Autodesk Inventor part; units mm, degrees
ref_plane "YZ Plane" through (0, 0, 0) normal (1, 0, 0) x (0, 1, 0)
ref_plane "XZ Plane" through (0, 0, 0) normal (0, 1, 0) x (-1, 0, 0)
ref_plane "XY Plane" through (0, 0, 0) normal (0, 0, 1) x (1, 0, 0)
sketch "Sketch1" plane through (0, 0, 0) normal (0, 0, 1) x (1, 0, 0)
  line L0 (0, 0) -> (-110.8614, 0)
  line L1 (-110.8614, 0) -> (-110.8614, -1490)
  line L2 (-110.8614, -1490) -> (0, -1490)
  line L3 (0, -1490) -> (0, 0)
  line L4 (-110.8614, -1390) -> (-66, -1390)
  line L5 (-66, -1390) -> (-66, -1385)
  line L6 (-66, -1385) -> (-110.8614, -1385)
  line L7 (-110.8614, -1385) -> (-110.8614, -1390)
  line L8 (-110.8614, -893.3333) -> (-66, -893.3333)
  line L9 (-66, -893.3333) -> (-66, -888.3333)
  line L10 (-66, -888.3333) -> (-110.8614, -888.3333)
  line L11 (-110.8614, -888.3333) -> (-110.8614, -893.3333)
  line L12 (-110.8614, -396.6667) -> (-66, -396.6667)
  line L13 (-66, -396.6667) -> (-66, -391.6667)
  line L14 (-66, -391.6667) -> (-110.8614, -391.6667)
  line L15 (-110.8614, -391.6667) -> (-110.8614, -396.6667)
  circle A0 centre (-110.8614, -155) radius 30
  point P0 (-110.8614, -1385)
  point P1 (-110.8614, -125)
  point P2 (-110.8614, -185)
  dimension "d0" = 1490
  dimension "d1" = 110.8614
  dimension "d2" = 5
  dimension "d4" = 100
  dimension "d7" = 496.6667
  dimension "d23" = 66
  dimension "d28" = 60
  dimension "d29" = 1335
extrude "Plate1" add sketch "Sketch1" along normal blind 4 contours L3 L2 L1 L4 L5 L6 L8 L9 L10 L12 L13 L14 A0 L0
sketch "Sketch2" plane through (4, 0, 0) normal (-1, 0, 0) x (0, -1, 0)
  line L0 (1490, 0) -> (0, 0)
  line L1 (0, 0) -> (0, 60)
  line L2 (0, 60) -> (1490, 60)
  line L3 (1490, 60) -> (1490, 0)
edge flange "Flange1" height 60 angle 90 thickness 4 bend radius 4 thickness toward (-1, 0, 0) relief tear relief width 4 relief depth 2 edges at (0, -745, 4) wall of the first edge with corners at (4, -1490, 0) (4, 0, 0) (4, 0, 60) (4, -1490, 60)
bend "Bend1"
corner "Corner1"
chamfer "Corner Chamfer1" distance 3 angle 45 6 edges at (-110.8614, -1390, 2) (-110.8614, -1385, 2) (-110.8614, -893.3333, 2) (-110.8614, -888.3333, 2) (-110.8614, -391.6667, 2) (-110.8614, -396.6667, 2)
equation "\"d0\" = Стрингер_длина"
equation "\"d1\" = стрингер_глубина_8"
equation "\"d2\" = паз_под_стрингер_толщина"
equation "\"d7\" = 0.333333 * Стрингер_длина"
equation "\"d23\" = паз_под_стрингер_глубина - Thickness"
equation "\"d28\" = 2 * радиус_выреза_под_сварку"
equation "\"d12\" = Thickness"
equation "\"d13\" = BendReliefWidth"
equation "\"d14\" = BendReliefDepth"
equation "\"d15\" = MinimumRemnant"
equation "\"d16\" = TransitionRadius"
equation "\"d17\" = ребро_усилителей"
equation "\"d19\" = BendRadius"
equation "\"d20\" = CornerReliefSize"
equation "\"d21\" = GapSize"
equation "\"d22\" = JacobiRadiusSize"
equation "\"BendRadius\" = Thickness"
equation "\"BendReliefWidth\" = Thickness"
equation "\"BendReliefDepth\" = 0.5 * Thickness"
equation "\"CornerReliefSize\" = 4 * Thickness"
equation "\"MinimumRemnant\" = 2 * Thickness"
equation "\"TransitionRadius\" = BendRadius"
equation "\"JacobiRadiusSize\" = BendRadius"
equation "\"GapSize\" = Thickness"
properties part number "0382 GBK stringer 8" material "Steel"
The model under review builds one solid part; all positions refer to its coordinate system, in mm. A direction names the side the tool comes from. Round coordinates to 2 decimals unless told otherwise and drop trailing zeros. Write each loop counter-clockwise with the first axis right and the second up, starting at its lowest first coordinate (ties: lowest second). Pieces come first, ordered by that corner, then holes. Notation, with made-up numbers: (12, 37.5) -> (51, 37.5) arc R24 ccw to (51, 68.5) -> close; hole circle Ø9 at (68, -29). An arc over 180 degrees is marked (long way). Use CSV: the item, a comma, the result in double quotes.
Q1. Consider section D-D (y = -155). Give the boundary of the cut face in (x, z), then the cut area to 3 significant figures.
Checks:
outline,"(-80.86, 0) -> (-4, 0) arc R8 ccw to (4, 8) -> (4, 60) -> (0, 60) -> (0, 8) arc R4 cw to (-4, 4) -> (-80.86, 4) -> close"
area,"553 mm²"
Q2. To check wall thickness, follow probe 1 along X at (y, z) = (-1242, 29). State the ranges of the line that lie inside material, in increasing order. Write a range as [from, to].
Checks:
probe 1,"[0, 4]"
Q3. Mouldability with a two-part tool opening along Y and no side actions: class faces 1 (the cylindrical face through (-80.87, -154.34, 1.97)), 2 (the flat face through (0, -735, 34)), 3 (the flat face through (-36, 0, 3)) as released by +Y, released by -Y, zero draft, split by the parting line, or undercut.
Checks:
face 1,"undercut"
face 2,"zero draft"
face 3,"released by +Y"
Q4. Consider section B-B (x = -37). Give the boundary of the cut face in (y, z).
Checks:
outline,"(-1490, 0) -> (0, 0) -> (0, 4) -> (-1490, 4) -> close"
Q5. For faces 4 (the flat face through (-58, -735, 4)), 5 (the flat face through (4, -735, 34)), list the 3-axis set-ups (+Z, -Z, +X, -X, +Y, -Y) from which the entire face can be reached by the end or side of a thin tool; tool diameter is ignored.
Checks:
face 4,"+Z, -X, +Y, -Y"
face 5,"+Z, -Z, +X, +Y, -Y"
Q6. Consider section C-C (z = 31.5). Give the boundary of the cut face in (x, y), then the cut area to 3 significant figures.
Checks:
outline,"(0, -1490) -> (4, -1490) -> (4, 0) -> (0, 0) -> close"
area,"5,960 mm²"
Q7. Consider section A-A (y = -649). Give the boundary of the cut face in (x, z), then the cut area to 3 significant figures.
Checks:
outline,"(-110.86, 0) -> (-4, 0) arc R8 ccw to (4, 8) -> (4, 60) -> (0, 60) -> (0, 8) arc R4 cw to (-4, 4) -> (-110.86, 4) -> close"
area,"673 mm²"
Q8. For pin 1 Ø4.5 at (y, z) = (-394, 2.5) entering from -X; pin 2 Ø6 at (x, y) = (-90.5, -842) entering from +Z; pin 3 Ø3 at (y, z) = (-795, 16.5) entering from -X, all flat-tipped, find the tip position at first contact; note any pin that passes through.
Checks:
pin 1,"x = -66"
pin 2,"z = 4"
pin 3,"x = 0"
